The model under review builds one solid part; all positions refer to its coordinate system, in mm. Face numbers are marked on the shaded views. Coordinates: 2 decimals unless noted, no trailing zeros. Write each loop counter-clockwise with the first axis right and the second up, starting at its lowest first coordinate (ties: lowest second). Pieces come first, ordered by that corner, then holes. Notation, with made-up numbers: (88, -19) - (146, -19) arc R20 cw to (146, 8) - close; hole circle Ø7 at (27.5, 74). An arc over 180 degrees is marked (long way). Put each result on its own line as item: value.
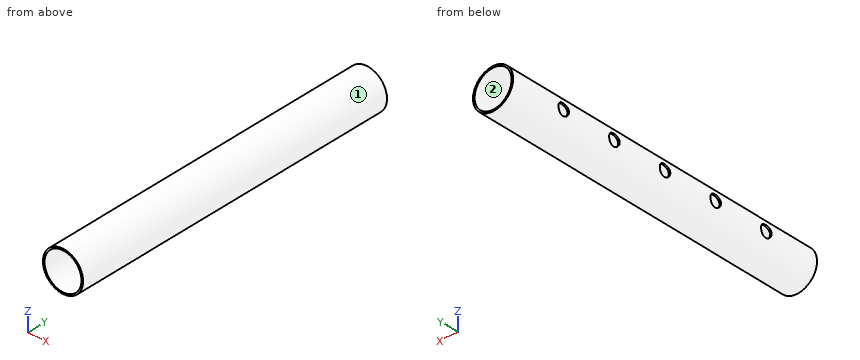
from build123d import *

# Parameters (mm, degrees)
F0_R     = 55.11276
F1_DEPTH = 914.4
F3_D     = 101.6
F5_R     = 15.875
F6_DEPTH = 88.9


with BuildPart() as f1:
    # F0 (on Front) → F1 (new body)
    with BuildSketch(Plane.XZ):
        Circle(F0_R)
    extrude(amount=F1_DEPTH)

    # F3 (through all)
    with Locations(Plane.XZ.offset(914.4)):
        with Locations((0, 0)):
            Hole(F3_D / 2)

    # F5 (on Right) → F6 (cut)
    with BuildSketch(Plane.YZ):
        with Locations((-762, 0)):
            Circle(F5_R)
        with Locations((-609.6, 0)):
            Circle(F5_R)
        with Locations((-457.2, 0)):
            Circle(F5_R)
        with Locations((-304.8, 0)):
            Circle(F5_R)
        with Locations((-152.4, 0)):
            Circle(F5_R)
    extrude(amount=-F6_DEPTH, mode=Mode.SUBTRACT)


solid = f1.part
1. Consider section A-A on x = 0. State the section outline as (y, z) points.
Determined:
outline: (-914.4, -55.11) - (0, -55.11) - (0, -50.8) - (-914.4, -50.8) - close; (-914.4, 50.8) - (0, 50.8) - (0, 55.11) - (-914.4, 55.11) - close
2. To check wall thickness, follow probe 1 along Y at (x, z) = (-53, 0) (3 decimals); probe 2 along X at (y, z) = (-789, 4); probe 3 along Z at (x, y) = (-50.5, -609.6) (3 decimals). State the ranges of each line that lie inside material, in increasing order.
Determined:
probe 1: y = -914.4 to -777.875, -746.125 to -625.475, -593.725 to -473.075, -441.325 to -320.675, -288.925 to -168.275, -136.525 to 0
probe 2: x = -54.97 to -50.64, 50.64 to 54.97
probe 3: z = -22.072 to -15.875, 15.875 to 22.072
3. Consider section C-C on y = -787.5. State the section outline as (x, z) points.
Determined:
outline: circle Ø110.23 at (0, 0); hole circle Ø101.6 at (0, 0)
4. The part is to be moulded in two halves that separate along X. For the marked faces 1 and 2, say which applies: +X half, -X half, draft (parallel to the pull), parting line (faces both ways), or undercut.
Determined:
face 1: parting line
face 2: undercut
5. For pin 1 Ø1 at (y, z) = (-165.5, -38) entering from +X; pin 2 Ø5 at (x, y) = (19.5, -469.5) entering from +Z; pin 3 Ø1.5 at (x, y) = (-16, -489) entering from -Z, all flat-tipped, find the tip position at first contact; note any pin that passes through.
Determined:
pin 1: stops at x = 40.39
pin 2: stops at z = 52.43
pin 3: stops at z = -52.96
6. Consider section B-B on z = 27. State the section outline as (x, y) points.
Determined:
outline: (-48.05, -914.4) - (-43.03, -914.4) - (-43.03, 0) - (-48.05, 0) - close; (43.03, -914.4) - (48.05, -914.4) - (48.05, 0) - (43.03, 0) - close
